from build123d import *

# Parameters (mm, degrees)
SFAZOWANIE1_SIZE = 1


with BuildPart() as part:
    # Szkic1 → Obrót1 (revolve)
    with BuildSketch(Plane.XY, mode=Mode.PRIVATE) as obr_t1_sk:
        with BuildLine():
            Line((0, 111.071464226), (-23.45, 111.071464226))
            Line((-23.45, 111.071464226), (-23.45, -18.141136369))
            ThreePointArc((-23.45, -18.141136369), (-23.824842317, -22.868718444), (-24.940002152, -27.478160664))
            Line((-24.940002152, -27.478160664), (-29.503332616, -41.411994143))
            ThreePointArc((-29.503332616, -41.411994143), (-29.875052561, -42.948474884), (-30, -44.524335575))
            Line((-30, -44.524335575), (-30, -48.928535774))
            Line((-30, -48.928535774), (-5, -48.928535774))
            Line((-5, -48.928535774), (-5, -45.928535774))
            Line((-5, -45.928535774), (0, -45.928535774))
            Line((0, -45.928535774), (0, 111.071464226))
        make_face()
    revolve(obr_t1_sk.sketch.rotate(Axis((0, -45.928535774, 0), (0, 1, 0)), 180), axis=Axis((0, -45.928535774, 0), (0, 1, 0)))

    # Sfazowanie1
    sfazowanie1_edges = [part.edges().sort_by_distance(p)[0] for p in [
        (-5, -48.928535774, 0),
        (-30, -48.928535774, 0),
    ]]
    chamfer(sfazowanie1_edges, length=SFAZOWANIE1_SIZE)


solid = part.part
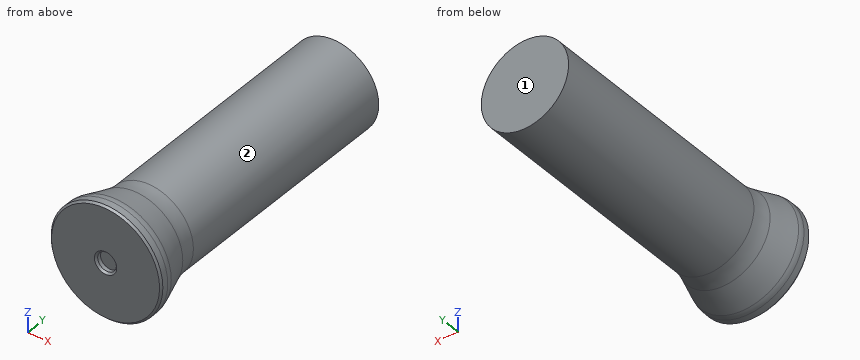
Work out the finished part from the listing and answer in its coordinate system (mm). Face numbers are marked on the shaded views. A direction names the side the tool comes from. Give positions to 0.01 mm unless a question says otherwise; leave off trailing zeros. Loops run counter-clockwise (first coordinate to the right, second up) from the corner with the lowest first, then second, coordinate; pieces in that order, holes last. Notation, with made-up numbers: (-31, 74.5) - (14, 74.5) arc R23 cw to (14, 98.5) - close; hole circle Ø7 at (10.5, -17). An arc over 180 degrees is marked (long way). Answer in a Markdown table with one row per item.
(1) Section B-B (x = 0) is taken. Give the vertices of the cut face in (y, z).
Results list:
| item | result |
|---|---|
| outline | (-48.93, -29) - (-47.93, -30) - (-44.52, -30) arc R10 ccw to (-41.41, -29.5) - (-27.48, -24.94) arc R30 cw to (-18.14, -23.45) - (111.07, -23.45) - (111.07, 23.45) - (-18.14, 23.45) arc R30 cw to (-27.48, 24.94) - (-41.41, 29.5) arc R10 ccw to (-44.52, 30) - (-47.93, 30) - (-48.93, 29) - (-48.93, 6) - (-47.93, 5) - (-45.93, 5) - (-45.93, -5) - (-47.93, -5) - (-48.93, -6) - close |
(2) Section A-A (z = 0) is taken. Give the vertices of the cut face in (x, y).
Results list:
| item | result |
|---|---|
| outline | (-30, -47.93) - (-29, -48.93) - (-6, -48.93) - (-5, -47.93) - (-5, -45.93) - (5, -45.93) - (5, -47.93) - (6, -48.93) - (29, -48.93) - (30, -47.93) - (30, -44.52) arc R10 ccw to (29.5, -41.41) - (24.94, -27.48) arc R30 cw to (23.45, -18.14) - (23.45, 111.07) - (-23.45, 111.07) - (-23.45, -18.14) arc R30 cw to (-24.94, -27.48) - (-29.5, -41.41) arc R10 ccw to (-30, -44.52) - close |
(3) A tool of negligible diameter and unlimited length cuts with its end or side. For the marked faces 1 and 2, from which of +Z, -Z, +X, -X, +Y, -Y can it reach the whole face along a straight path? Write none if from no direction.
Results list:
| item | result |
|---|---|
| face 1 | +Z, -Z, +X, -X, +Y |
| face 2 | +Y |
(4) Consider L1, parallel to Z at x = 0, y = -46.95; L2, parallel to Y at x = 2.5, z = 2; L3, parallel to Z at x = -12.5, y = 5. Determine where each line is inside the solid, lowest interval first. Write a range as [from, to].
Results list:
| item | result |
|---|---|
| L1 | z = [-30, -5], [5, 30] |
| L2 | y = [-45.93, 111.07] |
| L3 | z = [-19.84, 19.84] |
(5) Section D-D (y = -31) is taken. Give the vertices of the cut face in (x, z).
Results list:
| item | result |
|---|---|
| outline | circle Ø52.19 at (0, 0) |
(6) Flat-ended cylindrical pins translate along their axes: pin 1 Ø8 at (y, z) = (-23.5, 17) entering from +X; pin 2 Ø2 at (y, z) = (-24.5, -18.5) entering from +X; pin 3 Ø2 at (x, y) = (17.5, 32) entering from +Z. Find the tip coordinate at first contact, or state that the pin passes through.
Results list:
| item | result |
|---|---|
| pin 1 | stops at x = 20.28 |
| pin 2 | stops at x = 16.66 |
| pin 3 | stops at z = 16.66 |
(7) Section C-C (y = 33) is taken. Give the vertices of the cut face in (x, z).
Results list:
| item | result |
|---|---|
| outline | circle Ø46.9 at (0, 0) |
